Can you work these out from the model? Positions are in its coordinate system, mm. A direction names the side the tool comes from. Give positions to 0.01 mm unless a question says otherwise; leave off trailing zeros. Write each loop counter-clockwise with the first axis right and the second up, starting at its lowest first coordinate (ties: lowest second). Pieces come first, ordered by that corner, then holes. Notation, with made-up numbers: M 4.25,49.5 L 43.25,49.5 A36 ccw 43.25,85.5 Z; hole C -21.75,32.25 d6. An arc over 180 degrees is marked long. Use CSV: the item, a comma, the result in double quotes. Start each with the question number.
Autodesk Inventor part; units mm, degrees
ref_plane "YZ Plane" through (0, 0, 0) normal (1, 0, 0) x (0, 1, 0)
ref_plane "XZ Plane" through (0, 0, 0) normal (0, 1, 0) x (-1, 0, 0)
ref_plane "XY Plane" through (0, 0, 0) normal (0, 0, 1) x (1, 0, 0)
sketch "Sketch1" plane through (0, 0, 0) normal (0, 0, 1) x (1, 0, 0)
  line L0 (0, 0) -> (101.6, 0) construction
  line L1 (101.6, 0) -> (101.6, 38.1) construction
  line L2 (101.6, 38.1) -> (0, 38.1) construction
  line L3 (0, 38.1) -> (0, 0) construction
  line L4 (0, 0) -> (19.05, 0)
  line L5 (101.6, 0) -> (82.55, 0)
  line L6 (25.4, 6.35) -> (25.4, 15.875)
  line L7 (38.1, 28.575) -> (63.5, 28.575)
  line L8 (76.2, 15.875) -> (76.2, 6.35)
  line L9 (66.675, 31.75) -> (34.925, 31.75)
  line L10 (22.225, 19.05) -> (22.225, 9.525)
  line L11 (15.875, 3.175) -> (0, 3.175)
  line L12 (101.6, 3.175) -> (85.725, 3.175)
  line L13 (79.375, 9.525) -> (79.375, 19.05)
  line L14 (0, 0) -> (0, 3.175)
  line L15 (101.6, 0) -> (101.6, 3.175)
  arc A0 (34.925, 31.75) -> (22.225, 19.05) centre (34.925, 19.05) ccw
  arc A1 (38.1, 28.575) -> (25.4, 15.875) centre (38.1, 15.875) ccw
  arc A2 (79.375, 19.05) -> (66.675, 31.75) centre (66.675, 19.05) ccw
  arc A3 (76.2, 15.875) -> (63.5, 28.575) centre (63.5, 15.875) ccw
  arc A4 (15.875, 3.175) -> (22.225, 9.525) centre (15.875, 9.525) ccw
  arc A5 (79.375, 9.525) -> (85.725, 3.175) centre (85.725, 9.525) ccw
  arc A6 (76.2, 6.35) -> (82.55, 0) centre (82.55, 6.35) ccw
  arc A7 (19.05, 0) -> (25.4, 6.35) centre (19.05, 6.35) ccw
  point P0 (25.4, 0)
  point P1 (76.2, 0)
  point P2 (25.4, 28.575)
  dimension "d0" = 101.6
  dimension "d1" = 38.1
  dimension "d2" = 25.4
  dimension "d3" = 25.4
  dimension "d4" = 28.575
  dimension "d5" = 3.175
  dimension "d6" = 3.175
  dimension "d7" = 12.7
  dimension "d8" = 6.35
  dimension "d9" = 6.35
  dimension "d10" = 6.35
extrude "Extrusion1" add sketch "Sketch1" along normal blind 25.4
sketch "Sketch2" plane through (0, 0, 0) normal (0, -1, 0) x (1, 0, 0)
  line L0 (0, 0) -> (19.05, 0)
  line L1 (19.05, 0) -> (19.05, 25.4)
  line L2 (0, 25.4) -> (19.05, 25.4)
  line L3 (0, 0) -> (0, 25.4)
  line L4 (82.55, 0) -> (101.6, 0)
  line L5 (101.6, 0) -> (101.6, 25.4)
  line L6 (82.55, 25.4) -> (101.6, 25.4)
  line L7 (82.55, 0) -> (82.55, 25.4)
  point P0 (12.7, 12.7)
  point P1 (88.9, 12.7)
  dimension "d13" = 12.7
  dimension "d14" = 12.7
  dimension "d15" = 12.7
  dimension "d16" = 12.7
hole "Hole1" at (12.7, 0, 12.7) at (88.9, 0, 12.7) direction (0, 1, 0) diameter 6.35 end through all
fillet "Fillet1" radius 3.175 4 edges at (101.6, 1.5875, 25.4) (101.6, 1.5875, 0) (0, 1.5875, 25.4) (0, 1.5875, 0)
properties part number "hendel"
(1) I want a section at D-D (z = 10.75). Write out the boundary of the cut face in (x, y) (3 decimals), and give its area (3 significant figures).
(2) I want a section at B-B (y = 11). Write out the boundary of the cut face in (x, z) (3 decimals).
(3) I want a section at C-C (z = 20.75). Write out the boundary of the cut face in (x, y) (3 decimals).
(4) Please list where these lines run through material, in increasing order: L1, parallel to Z at x = 88.9, y = 0.9 (3 decimals); L2, parallel to X at y = 10.5, z = 8.5 (3 decimals); L3, parallel to X at y = 1.8, z = 12.7 (3 decimals). Write a range as [from, to].
(5) Will these pins go through, and if not, where does the flat tip stop? pin 1 Ø1.5 at (x, z) = (68, 14.5) entering from +Y; pin 2 Ø7.5 at (x, z) = (12.7, 12.7) entering from -Y; pin 3 Ø8 at (x, z) = (7, 10) entering from +Y (3 decimals); pin 4 Ø6 at (y, z) = (12, 12) entering from -X.
(6) Which directions (+Z, -Z, +X, -X, +Y, -Y) give clear straight access to the entire face, cutting with the end or side of a thin tool? Please do faces 1 (the face through (23.59, 1.91, 12.52)), 2 (the face through (22.225, 14, 13)), 3 (the face through (94, 3.175, 13)).
(7) I want a section at A-A (x = 12.7). Write out the boundary of the cut face in (y, z) (3 decimals).
Geometry results:
1,outline,"M 0,0 L 10.194,0 L 10.194,3.175 L 0,3.175 Z; M 15.206,0 L 19.05,0 A6.35 ccw 25.4,6.35 L 25.4,15.875 A12.7 cw 38.1,28.575 L 63.5,28.575 A12.7 cw 76.2,15.875 L 76.2,6.35 A6.35 ccw 82.55,0 L 86.394,0 L 86.394,3.175 L 85.725,3.175 A6.35 cw 79.375,9.525 L 79.375,19.05 A12.7 ccw 66.675,31.75 L 34.925,31.75 A12.7 ccw 22.225,19.05 L 22.225,9.525 A6.35 cw 15.875,3.175 L 15.206,3.175 Z; M 91.406,0 L 101.6,0 L 101.6,3.175 L 91.406,3.175 Z"
1,area,"472 mm2"
2,outline,"M 22.225,0 L 25.4,0 L 25.4,25.4 L 22.225,25.4 Z; M 76.2,0 L 79.375,0 L 79.375,25.4 L 76.2,25.4 Z"
3,outline,"M 0,0 L 19.05,0 A6.35 ccw 25.4,6.35 L 25.4,15.875 A12.7 cw 38.1,28.575 L 63.5,28.575 A12.7 cw 76.2,15.875 L 76.2,6.35 A6.35 ccw 82.55,0 L 101.6,0 L 101.6,3.175 L 85.725,3.175 A6.35 cw 79.375,9.525 L 79.375,19.05 A12.7 ccw 66.675,31.75 L 34.925,31.75 A12.7 ccw 22.225,19.05 L 22.225,9.525 A6.35 cw 15.875,3.175 L 0,3.175 Z"
4,L1,"z = [0, 9.525], [15.875, 25.4]"
4,L2,"x = [22.225, 25.4], [76.2, 79.375]"
4,L3,"x = [0, 9.525], [15.875, 23.479], [78.121, 85.725], [92.075, 101.6]"
5,pin 1,"stops at y = 31.74"
5,pin 2,"stops at y = 0"
5,pin 3,"stops at y = 3.175"
5,pin 4,"stops at x = 22.2"
6,face 1,"+Z, -Z, -Y"
6,face 2,"+Z, -Z, -X, +Y"
6,face 3,"+Z, -Z, +X, +Y"
7,outline,"M 0,0 L 3.175,0 L 3.175,9.525 L 0,9.525 Z; M 0,15.875 L 3.175,15.875 L 3.175,25.4 L 0,25.4 Z"
